Here's how the part is built. I have some questions about the finished solid (model axes, mm). A direction names the side the tool comes from. Give positions to 0.01 mm unless a question says otherwise; leave off trailing zeros. Order: outer loops, then holes, each group sorted by start corner. A loop starts at its lowest first (then second) coordinate and runs counter-clockwise, first axis right, second up. Notation, with made-up numbers: M -21.5,78 L -6.5,78 A31 ccw -6.5,104 Z; hole C 5,-37.5 d6. An arc over 180 degrees is marked long. Use one line per item in the form item = value.
from build123d import *

# Parameters (mm, degrees)
SKETCH1_W           = 20
SKETCH1_H           = 5.5
BOSS_EXTRUDE1_DEPTH = 5


with BuildPart() as part:
    # Sketch1 → Boss-Extrude1 (new body)
    with BuildSketch(Plane.XY):
        with BuildLine():
            Line((-112, 0), (-95, 0))
            Line((-95, 0), (-95, 17))
            Line((-95, 17), (-95, 35))
            ThreePointArc((-95, 35), (-86.213203436, 56.213203436), (-65, 65))
            Line((-65, 65), (-55, 65))
            Line((-55, 65), (55, 65))
            Line((55, 65), (95, 17))
            Line((95, 17), (95, 0))
            Line((95, 0), (112, 0))
            Line((112, 0), (112, 21))
            Line((112, 21), (61.166666667, 82))
            Line((61.166666667, 82), (-61.166666667, 82))
            Line((-61.166666667, 82), (-62, 82))
            ThreePointArc((-62, 82), (-97.355339059, 67.355339059), (-112, 32))
            Line((-112, 32), (-112, 21))
            Line((-112, 21), (-112, 0))
        make_face()
        with Locations((29, 73.5)):
            Rectangle(SKETCH1_W, SKETCH1_H, mode=Mode.SUBTRACT)
        with Locations((-29, 73.5)):
            Rectangle(SKETCH1_W, SKETCH1_H, mode=Mode.SUBTRACT)
    extrude(amount=BOSS_EXTRUDE1_DEPTH)


solid = part.part
Q1. I want a section at D-D on x = -54. Write out the boundary of the cut face in (y, z).
Found:
outline = M 65,0 L 82,0 L 82,5 L 65,5 Z
Q2. On a 3-axis mill with a long thin cutter (end or side, diameter ignored), from which of +Z, -Z, +X, -X, +Y, -Y can I reach the whole of each face in a straight line? I mean faces 1 (the face through (29, 76.25, 2)), 2 (the face through (75, 41, 2)), 3 (the face through (-96.964, 67.742, 2.465)). Say none if no direction works.
Found:
face_1 = +Z, -Z
face_2 = +Z, -Z, -Y
face_3 = +Z, -Z, -X, +Y
Q3. I'm going to push a flat-ended pin straight in: pin 1 Ø1.5 at (y, z) = (73.5, 1.5) entering from +X (3 decimals). Where does the tip first touch, or does it pass through?
Found:
pin_1 = 68.875
Q4. I want a section at C-C on y = 27.5. Write out the boundary of the cut face in (x, z).
Found:
outline = M -112,0 L -95,0 L -95,5 L -112,5 Z; M 86.25,0 L 106.58,0 L 106.58,5 L 86.25,5 Z
Q5. I want a section at A-A on x = -23. Write out the boundary of the cut face in (y, z), then the cut area to 3 significant figures.
Found:
outline = M 65,0 L 70.75,0 L 70.75,5 L 65,5 Z; M 76.25,0 L 82,0 L 82,5 L 76.25,5 Z
area = 57.5 mm²
Q6. Thinking about a two-plate mould opening in X: for faces 4 (the face through (112, 10, 2)), 5 (the face through (-104, 0, 2)), 6 (the face through (-19, 73, 2)), which applies, +X half, -X half, draft (parallel to the pull), parting line (faces both ways), or undercut?
Found:
face_4 = +X half
face_5 = draft
face_6 = undercut
Q7. I need wall thicknesses on L1, parallel to Y at x = -24, z = 1.95; L2, parallel to X at y = 8.5, z = 0.35; L3, parallel to X at y = 55.5, z = 2.7. Which ranges of each line are inside material? Lowest first, please.
Found:
L1 = 65 to 70.75, 76.25 to 82
L2 = -112 to -95, 95 to 112
L3 = -106.13 to -86.9, 62.92 to 83.25
Q8. I want a section at B-B on z = 3. Write out the boundary of the cut face in (x, y), then the cut area to 3 significant figures.
Found:
outline = M -112,0 L -95,0 L -95,35 A30 cw -65,65 L 55,65 L 95,17 L 95,0 L 112,0 L 112,21 L 61.17,82 L -62,82 A50 ccw -112,32 Z; hole M -39,70.75 L -19,70.75 L -19,76.25 L -39,76.25 Z; hole M 19,70.75 L 39,70.75 L 39,76.25 L 19,76.25 Z
area = 4,860 mm²
